Design review of the part built by this model. Coordinates are the model's own, in mm. A direction names the side the tool comes from. Coordinates: 2 decimals unless noted, no trailing zeros. Loops run counter-clockwise (first coordinate to the right, second up) from the corner with the lowest first, then second, coordinate; pieces in that order, holes last. Notation, with made-up numbers: (-21, 9.25) -> (4, 9.25) arc R9 cw to (4, 21.25) -> close; hole circle Ø7 at (-14, -38.5). An arc over 180 degrees is marked (long way). Answer in a Markdown table with one row per item.
```python
from build123d import *

# Parameters (mm, degrees)
F0_W     = 6.35
F0_H     = 12.7
F1_DEPTH = 25.4
F2_R     = 6.34999
F3_R     = 3.175
F4_DEPTH = 3.175


# Not quite as in the source:
# - a fillet or chamfer is up to 0.001 mm smaller than in the source, because OpenCascade refuses the exact size


with BuildPart() as f1:
    # F0 (on Front) → F1 (new body)
    with BuildSketch(Plane.XZ):
        Rectangle(F0_W, F0_H)
    extrude(amount=F1_DEPTH)

    # F2 (radius 6.35 in the source; OpenCascade refuses exactly that, so slightly less here)
    f2_edges = [f1.edges().sort_by_distance(p)[0] for p in [
        (0, -25.4, 6.35),
        (0, -25.4, -6.35),
    ]]
    fillet(f2_edges, radius=F2_R)

    # F3 (on face) → F4 (cut)
    with BuildSketch(Plane(origin=(-3.175, 0, 0), x_dir=(0, -1, 0), z_dir=(-1, 0, 0))):
        with Locations((19.05, 0)):
            Circle(F3_R)
    extrude(amount=-F4_DEPTH, mode=Mode.SUBTRACT)


solid = f1.part
```
(1) Take a section at D-D on z = 2. Give the boundary of the cut face in (x, y) (3 decimals).
Evaluation:
| item | result |
|---|---|
| outline | (-3.175, -25.077) -> (3.175, -25.077) -> (3.175, 0) -> (-3.175, 0) -> (-3.175, -16.584) -> (0, -16.584) -> (0, -21.516) -> (-3.175, -21.516) -> close |
(2) For pin 1 (7.5 mm diameter, centred on y = -19.05, z = 0, fed in from -X) (3 decimals); pin 2 (1.9 mm diameter, centred on y = -19, z = -1.5, fed in from -X); pin 3 (1 mm diameter, centred on x = 0.5, z = 1.5, fed in from -Y), all flat-tipped, find the tip position at first contact; note any pin that passes through.
Evaluation:
| item | result |
|---|---|
| pin 1 | stops at x = -3.175 |
| pin 2 | stops at x = 0 |
| pin 3 | stops at y = -25.32 |
(3) Draft analysis for pull direction Z (two halves, no side actions). For faces 3 (the flat face through (-3.175, -13, 0)), 4 (the flat face through (0, -9, 6.35)), 5 (the flat face through (0, -19, 0)), state which applies: pulls with the +Z half, pulls with the -Z half, needs draft (parallel to the pull), parting line crosses it, or undercut.
Evaluation:
| item | result |
|---|---|
| face 3 | needs draft |
| face 4 | pulls with the +Z half |
| face 5 | undercut |
(4) Tool access review of faces 1 (the flat face through (0, 0, 0)), 2 (the cylindrical face through (-1.61, -15.88, 0.14)): name each direction out of +Z, -Z, +X, -X, +Y, -Y from which nothing blocks a thin tool from reaching the whole face with its end or side.
Evaluation:
| item | result |
|---|---|
| face 1 | +Z, -Z, +X, -X, +Y |
| face 2 | -X |
(5) To check wall thickness, follow probe 1 along Z at (x, y) = (-1, -19.05) (3 decimals); probe 2 along Y at (x, z) = (-0.75, -1); probe 3 along Y at (x, z) = (1, 5.5). State the ranges of each line that lie inside material, in increasing order.
Evaluation:
| item | result |
|---|---|
| probe 1 | z = -6.35 to -3.175, 3.175 to 6.35 |
| probe 2 | y = -25.32 to -22.06, -16.04 to 0 |
| probe 3 | y = -22.22 to 0 |
(6) Take a section at B-B on y = -21.25. Give the boundary of the cut face in (x, z) (3 decimals), and give its area (3 significant figures).
Evaluation:
| item | result |
|---|---|
| outline | (-3.175, -5.957) -> (3.175, -5.957) -> (3.175, 5.957) -> (-3.175, 5.957) -> (-3.175, 2.289) -> (0, 2.289) -> (0, -2.289) -> (-3.175, -2.289) -> close |
| area | 61.1 mm² |
